Read the model definition and answer for the solid it produces. Units are mm, in the model's axes. A direction names the side the tool comes from. Coordinates: 2 decimals unless noted, no trailing zeros. Loops run counter-clockwise (first coordinate to the right, second up) from the corner with the lowest first, then second, coordinate; pieces in that order, holes last. Notation, with made-up numbers: M 43,-4 L 82,-4 A26 ccw 82,18 Z; hole C -19.5,74 d3. An arc over 180 degrees is marked long. Use one line per item in the form item = value. Start each with the question number.
1. For a pull along Z with two mould halves and no side action, classify faces 1 (the flat face through (22, 4, -18)), 2 (the cylindrical face through (1.141, 5.324, -38.797)), 3 (the cylindrical face through (8.89, 1.01, -22.22)), 4 (the flat face through (11, 12, 0)) as released by +Z, released by -Z, zero draft, split by the parting line, or undercut.
2. A tool of negligible diameter and unlimited length cuts with its end or side. For faces 5 (the flat face through (18, 10.5, -21)), 6 (the flat face through (11, 8, -8)), 7 (the flat face through (0, 4, -18)), from which of +Z, -Z, +X, -X, +Y, -Y can it reach the whole face along a straight path? Write none if from no direction.
3. Find the intervals of material crossed by probe 1 along Y at (x, z) = (11, -1.05) (3 decimals); probe 2 along X at (y, z) = (9, -35.5); probe 3 along Y at (x, z) = (3.75, -11.5), in increasing order. Write a range as [from, to].
4. The part is cut by section D-D (y = 20.5). Give the vertices of the cut face in (x, z).
5. The part is cut by section C-C (z = -27.3). Give the vertices of the cut face in (x, y), plus the area to 3 significant figures.
6. The part is cut by section B-B (y = 18). Give the vertices of the cut face in (x, z) (3 decimals), plus the area to 3 significant figures.
7. Flat-ended cylindrical pins translate along their axes: pin 1 (6.5 mm diameter, centred on x = 11, z = -27.3, fed in from -Y); pin 2 (0.7 mm diameter, centred on x = 11, z = -7.5, fed in from +Y); pin 3 (5 mm diameter, centred on x = 13.5, z = -16.5, fed in from +Y); pin 4 (2 mm diameter, centred on x = 4.275, y = 18, fed in from -Z). Find the tip coordinate at first contact, or state that the pin passes through.
8. The part is cut by section A-A (x = 11). Give the vertices of the cut face in (y, z) (3 decimals).
from build123d import *

# Parameters (mm, degrees)
SKETCH1_W           = 22
SKETCH1_H           = 40
BOSS_EXTRUDE1_DEPTH = 10.5
SKETCH2_W           = 13
SKETCH2_H           = 23
CUT_EXTRUDE1_DEPTH  = 8.5
SKETCH3_R           = 5.5
CUT_EXTRUDE2_DEPTH  = 47.435439053
SKETCH4_W           = 22
SKETCH4_H           = 1.7
BOSS_EXTRUDE2_DEPTH = 14
SKETCH5_R           = 3.725
CUT_EXTRUDE3_DEPTH  = 51.508811113
SKETCH5_3_R         = 3.725
SKETCH5_3_R_2       = 0.7
CUT_EXTRUDE4_DEPTH  = 10
SKETCH6_R           = 0.7
CUT_EXTRUDE5_DEPTH  = 2.5
FILLET1_R           = 4
FILLET2_R           = 2.5


with BuildPart() as part:
    # Sketch1 → Boss-Extrude1 (new body)
    with BuildSketch(Plane(origin=(0, 0, 0), x_dir=(1, 0, 0), z_dir=(0, 1, 0))):
        with Locations((11, 20)):
            Rectangle(SKETCH1_W, SKETCH1_H)
    extrude(amount=BOSS_EXTRUDE1_DEPTH)

    # Sketch2 → Cut-Extrude1 (cut)
    with BuildSketch(Plane(origin=(0, 10.5, 0), x_dir=(1, 0, 0), z_dir=(0, 1, 0))):
        with Locations((11, 22)):
            Rectangle(SKETCH2_W, SKETCH2_H)
    extrude(amount=-CUT_EXTRUDE1_DEPTH, mode=Mode.SUBTRACT)

    # Sketch3 → Cut-Extrude2 (cut, through all)
    with BuildSketch(Plane(origin=(0, 2, 0), x_dir=(1, 0, 0), z_dir=(0, 1, 0))):
        with Locations(Location((11, 27.3, 0), (0, 0, 270))):
            Circle(SKETCH3_R)
    extrude(amount=-CUT_EXTRUDE2_DEPTH, mode=Mode.SUBTRACT)

    # Sketch4 → Boss-Extrude2 (add)
    with BuildSketch(Plane(origin=(0, 10.5, 0), x_dir=(1, 0, 0), z_dir=(0, 1, 0))):
        with Locations((11, 0.85)):
            Rectangle(SKETCH4_W, SKETCH4_H)
    extrude(amount=BOSS_EXTRUDE2_DEPTH)

    # Sketch5 → Cut-Extrude3 (cut, through all)
    with BuildSketch(Plane(origin=(0, 0, -1.7), x_dir=(-1, 0, 0), z_dir=(0, 0, -1))):
        with Locations((-11, 18)):
            Circle(SKETCH5_R)
    extrude(amount=-CUT_EXTRUDE3_DEPTH, mode=Mode.SUBTRACT)

    # Sketch5_3 → Cut-Extrude4 (cut)
    with BuildSketch(Plane(origin=(0, 0, -1.7), x_dir=(-1, 0, 0), z_dir=(0, 0, -1))):
        with Locations((-11, 18)):
            Circle(SKETCH5_3_R)
        with Locations((-17.725, 18)):
            Circle(SKETCH5_3_R_2)
        with Locations((-4.275, 18)):
            Circle(SKETCH5_3_R_2)
    extrude(amount=-CUT_EXTRUDE4_DEPTH, mode=Mode.SUBTRACT)

    # Sketch6 → Cut-Extrude5 (cut)
    with BuildSketch(Plane(origin=(0, 10.5, 0), x_dir=(1, 0, 0), z_dir=(0, 1, 0))):
        with Locations(Location((11, 35.5, 0), (0, 0, 270))):
            Circle(SKETCH6_R)
        with Locations(Location((11, 7.5, 0), (0, 0, 270))):
            Circle(SKETCH6_R)
    extrude(amount=-CUT_EXTRUDE5_DEPTH, mode=Mode.SUBTRACT)

    # Fillet1
    fillet1_edges = [part.edges().sort_by_distance(p)[0] for p in [
        (0, 5.25, -40),
        (22, 5.25, -40),
    ]]
    fillet(fillet1_edges, radius=FILLET1_R)

    # Fillet2
    fillet2_edges = [part.edges().sort_by_distance(p)[0] for p in [
        (0, 24.5, -0.85),
        (22, 24.5, -0.85),
    ]]
    fillet(fillet2_edges, radius=FILLET2_R)


solid = part.part
Computed values:
q1.face_1 = zero draft
q1.face_2 = released by -Z
q1.face_3 = undercut
q1.face_4 = released by +Z
q2.face_5 = -Z, +X, -X, +Y
q2.face_6 = +Y
q2.face_7 = +Z, -Z, -X, +Y, -Y
q3.probe_1 = [0, 14.275], [21.725, 24.5]
q3.probe_2 = [0, 10.3], [11.7, 22]
q3.probe_3 = [0, 10.5]
q4.outline = M 0,-1.7 L 8.24,-1.7 L 8.24,0 L 0,0 Z; M 13.76,-1.7 L 22,-1.7 L 22,0 L 13.76,0 Z
q5.outline = M 0,0 L 5.5,0 L 5.5,2 L 4.5,2 L 4.5,10.5 L 0,10.5 Z; M 16.5,0 L 22,0 L 22,10.5 L 17.5,10.5 L 17.5,2 L 16.5,2 Z
q5.area = 98.5 mm²
q6.outline = M 0,-1.7 L 3.575,-1.7 L 3.575,0 L 0,0 Z; M 4.975,-1.7 L 7.275,-1.7 L 7.275,0 L 4.975,0 Z; M 14.725,-1.7 L 17.025,-1.7 L 17.025,0 L 14.725,0 Z; M 18.425,-1.7 L 22,-1.7 L 22,0 L 18.425,0 Z
q6.area = 20.0 mm²
q7.pin_1 = through
q7.pin_2 = 8
q7.pin_3 = 2
q7.pin_4 = -1.7
q8.outline = M 0,-40 L 10.5,-40 L 10.5,-36.2 L 8,-36.2 L 8,-34.8 L 10.5,-34.8 L 10.5,-33.5 L 2,-33.5 L 2,-32.8 L 0,-32.8 Z; M 0,-21.8 L 2,-21.8 L 2,-10.5 L 10.5,-10.5 L 10.5,-8.2 L 8,-8.2 L 8,-6.8 L 10.5,-6.8 L 10.5,-1.7 L 14.275,-1.7 L 14.275,0 L 0,0 Z; M 21.725,-1.7 L 24.5,-1.7 L 24.5,0 L 21.725,0 Z
